Model file for the job. Use its own axes, mm. A direction names the side the tool comes from. Round coordinates to 2 decimals unless told otherwise and drop trailing zeros. Loops run counter-clockwise (first coordinate to the right, second up) from the corner with the lowest first, then second, coordinate; pieces in that order, holes last. Notation, with made-up numbers: M 8.5,59.5 L 56.5,59.5 A18 cw 56.5,79.5 Z; hole C -5,79 d6. An arc over 180 degrees is marked long. Use a Markdown table: item, result. Add a question column.
Item 1: Saw through at B-B on x = 20. Write the cut outline in (y, z).
Item 2: Two-plate mould, pull along Y, no slides. Class faces 4 (the flat face through (0, 0, 4)), 5 (the flat face through (7.95, -17, 2)), 6 (the flat face through (-6, 0, 0)), 7 (the flat face through (5.2, -6.55, 4.2)): +Y half, -Y half, draft (parallel to the pull), parting line (faces both ways), or undercut.
Item 3: Tool access for faces 1 (the flat face through (-7, 12.3, 2)), 2 (the flat face through (-24.5, 16, 2)), 3 (the flat face through (0, 2.55, 5)): list every direction of +Z, -Z, +X, -X, +Y, -Y with a clear straight run to the whole face (end or side of a thin tool).
Item 4: Saw through at A-A on y = 19. Write the cut outline in (x, z), then the cut area to 3 significant figures.
Item 5: Pin check, flat tips, straight feed: P1, Ø3, axis at x = 2.5, y = 0, coming from the +Z side; P2, Ø1.5, axis at x = 4.5, z = 6, coming from the -Y side; P3, Ø1.2, axis at y = -18.5, z = 3, coming from the +X side. Stop position of each tip, or through.
Item 6: Saw through at D-D on x = -6.5. Write the cut outline in (y, z).
Item 7: Saw through at C-C on z = 5.25. Write the cut outline in (x, y), then the cut area to 3 significant figures.
Item 8: Wall check: L1, parallel to Y at x = -13.5, z = 0.75; L2, parallel to Y at x = -13, z = 5.75; L3, parallel to Y at x = 20, z = 2.5. Give the ranges that are in metal, low to high. Write a range as from..to.
```python
from build123d import *

# Parameters (mm, degrees)
CROQUIS1_R              = 1.55
SALIENTE_EXTRUIR1_DEPTH = 4
CROQUIS2_W              = 50
CROQUIS2_H              = 4
SALIENTE_EXTRUIR2_DEPTH = 7
SALIENTE_EXTRUIR3_START = -7
CROQUIS3_W              = 34.5
CROQUIS3_H              = 21.5
CROQUIS3_R              = 1.55
CROQUIS3_W_2            = 29.9
CROQUIS3_H_2            = 10
SALIENTE_EXTRUIR3_DEPTH = 4
REDONDEO1_R             = 2
CHAFL_N1_SIZE           = 0.4


with BuildPart() as part:
    # Croquis1 → Saliente-Extruir1 (new body)
    # profile 1 of 3: a face of its own
    with BuildSketch(Plane.XY):
        with BuildLine():
            ThreePointArc((-20, 2.55), (-22.55, 0), (-20, -2.55))
            Line((-20, -2.55), (-25, -2.55))
            Line((-25, -2.55), (-25, 2.55))
            Line((-25, 2.55), (-20, 2.55))
        make_face()
    # profile 2 of 3: a face of its own
    with BuildSketch(Plane.XY):
        with BuildLine():
            Line((-20, -2.55), (20, -2.55))
            ThreePointArc((20, -2.55), (22.55, 0), (20, 2.55))
            Line((20, 2.55), (-20, 2.55))
            ThreePointArc((-20, 2.55), (-22.55, 0), (-20, -2.55))
        make_face()
        with Locations((-20, 0)):
            Circle(CROQUIS1_R, mode=Mode.SUBTRACT)
        with Locations((20, 0)):
            Circle(CROQUIS1_R, mode=Mode.SUBTRACT)
    # profile 3 of 3: a face of its own
    with BuildSketch(Plane.XY):
        with BuildLine():
            ThreePointArc((20, -2.55), (22.55, 0), (20, 2.55))
            Line((20, 2.55), (25, 2.55))
            Line((25, 2.55), (25, -2.55))
            Line((25, -2.55), (20, -2.55))
        make_face()
    extrude(amount=SALIENTE_EXTRUIR1_DEPTH)

    # Croquis2 → Saliente-Extruir2 (add)
    with BuildSketch(Plane.XY):
        with Locations((0, 4.55)):
            Rectangle(CROQUIS2_W, CROQUIS2_H)
        with Locations((0, -4.55)):
            Rectangle(CROQUIS2_W, CROQUIS2_H)
    extrude(amount=SALIENTE_EXTRUIR2_DEPTH)

    # Croquis3 → Saliente-Extruir3 (add)
    # profile 1 of 2: a face of its own
    with BuildSketch(Plane.XY.offset(7).offset(SALIENTE_EXTRUIR3_START)):
        with Locations((-7.25, 17.3)):
            Rectangle(CROQUIS3_W, CROQUIS3_H)
        with Locations((-21.95, 25.5)):
            Circle(CROQUIS3_R, mode=Mode.SUBTRACT)
        with Locations((7.95, 9.6)):
            Circle(CROQUIS3_R, mode=Mode.SUBTRACT)
        with Locations((-7, 17.3)):
            Rectangle(CROQUIS3_W_2, CROQUIS3_H_2, mode=Mode.SUBTRACT)
    # profile 2 of 2: a face of its own
    with BuildSketch(Plane.XY.offset(7).offset(SALIENTE_EXTRUIR3_START)):
        with Locations((-7.25, -17.3)):
            Rectangle(CROQUIS3_W, CROQUIS3_H)
        with Locations((-21.95, -9.1)):
            Circle(CROQUIS3_R, mode=Mode.SUBTRACT)
        with Locations((-7, -17.3)):
            Rectangle(CROQUIS3_W_2, CROQUIS3_H_2, mode=Mode.SUBTRACT)
        with Locations((7.95, -25)):
            Circle(CROQUIS3_R, mode=Mode.SUBTRACT)
    extrude(amount=SALIENTE_EXTRUIR3_DEPTH)

    # Redondeo1
    redondeo1_edges = [part.edges().sort_by_distance(p)[0] for p in [
        (-24.5, 28.05, 2),
        (10, 28.05, 2),
        (-24.5, -28.05, 2),
        (10, -28.05, 2),
    ]]
    fillet(redondeo1_edges, radius=REDONDEO1_R)

    # Chaflán1
    chafl_n1_edges = [part.edges().sort_by_distance(p)[0] for p in [
        (-23.5, 25.5, 4),
        (6.4, 9.6, 4),
        (-23.5, -9.1, 4),
        (6.4, -25, 4),
    ]]
    chamfer(chafl_n1_edges, length=CHAFL_N1_SIZE)


solid = part.part
```
Entries:
| question | item | result |
|---|---|---|
| 1 | outline | M -6.55,0 L -1.55,0 L -1.55,4 L -2.55,4 L -2.55,7 L -6.55,7 Z; M 1.55,0 L 6.55,0 L 6.55,7 L 2.55,7 L 2.55,4 L 1.55,4 Z |
| 2 | face 4 | undercut |
| 2 | face 5 | undercut |
| 2 | face 6 | draft |
| 2 | face 7 | -Y half |
| 3 | face 1 | +Z, -Z |
| 3 | face 2 | +Z, -Z, -X, +Y |
| 3 | face 3 | +Z, +X, -X |
| 4 | outline | M -24.5,0 L -21.95,0 L -21.95,4 L -24.5,4 Z; M 7.95,0 L 10,0 L 10,4 L 7.95,4 Z |
| 4 | area | 18.4 mm2 |
| 5 | P1 | z = 4 |
| 5 | P2 | y = -6.55 |
| 5 | P3 | x = 10 |
| 6 | outline | M -28.05,0 L -22.3,0 L -22.3,4 L -28.05,4 Z; M -12.3,0 L 12.3,0 L 12.3,4 L 6.55,4 L 6.55,7 L 2.55,7 L 2.55,4 L -2.55,4 L -2.55,7 L -6.55,7 L -6.55,4 L -12.3,4 Z; M 22.3,0 L 28.05,0 L 28.05,4 L 22.3,4 Z |
| 7 | outline | M -25,-6.55 L 25,-6.55 L 25,-2.55 L -25,-2.55 Z; M -25,2.55 L 25,2.55 L 25,6.55 L -25,6.55 Z |
| 7 | area | 400 mm2 |
| 8 | L1 | -28.05..-22.3, -12.3..12.3, 22.3..28.05 |
| 8 | L2 | -6.55..-2.55, 2.55..6.55 |
| 8 | L3 | -6.55..-1.55, 1.55..6.55 |
